Could you check a few things on this model? Use its own coordinates, in mm. A direction names the side the tool comes from. Round coordinates to 2 decimals unless told otherwise and drop trailing zeros. Write each loop counter-clockwise with the first axis right and the second up, starting at its lowest first coordinate (ties: lowest second). Pieces come first, ordered by that corner, then holes. Notation, with made-up numbers: M 51.5,-30 L 74.5,-30 A14 cw 74.5,-23 Z; hole C 60,51.5 d7. An arc over 180 degrees is marked long. One line per item, written item: value. Start each with the question number.
(1) If I drill on L1, parallel to Z at x = 8.89, y = 5; L2, parallel to Z at x = -0.5, y = 2.5; L3, parallel to Z at x = -19, y = 4.75, over which ranges is the centre line in solid material (lowest first)?
(2) I want a section at A-A on x = 0. Please give me the cut outline in (y, z).
(3) I want a section at B-B on z = 0. Please give me the cut outline in (x, y).
(4) I want a section at D-D on x = 5.5. Please give me the cut outline in (y, z), and give its area (3 significant figures).
(5) Which directions (+Z, -Z, +X, -X, +Y, -Y) give clear straight access to the entire face, cutting with the end or side of a thin tool? Please do faces 5 (the face through (-0.73, 3.13, -4.94)), 6 (the face through (15, 3, 15)), 7 (the face through (-20.047, 3.131, -5.372)).
(6) I'm going to push flat-ended pins straight in: pin 1 Ø2 at (y, z) = (2.5, 15) entering from +X; pin 2 Ø2 at (y, z) = (2.5, -13) entering from +X. Where does each tip first touch, or does it pass through?
(7) Thinking about a two-plate mould opening in X: for faces 1 (the face through (-9.06, 3.13, -15.3)), 2 (the face through (11.98, 3.13, 20.58)), 3 (the face through (2, 0, 0)), 4 (the face through (-23.812, 3.131, 0.087)), which applies, released by +X, released by -X, zero draft, split by the parting line, or undercut?
(8) I want a section at C-C on y = 5.25. Count the separate pieces of the cut face and the enclosed holes in it, and give its area (3 significant figures).
Autodesk Inventor part; units mm, degrees
ref_plane "YZ Plane" through (0, 0, 0) normal (1, 0, 0) x (0, 1, 0)
ref_plane "XZ Plane" through (0, 0, 0) normal (0, 1, 0) x (-1, 0, 0)
ref_plane "XY Plane" through (0, 0, 0) normal (0, 0, 1) x (1, 0, 0)
sketch "Sketch1" plane through (0, 0, 0) normal (0, 1, 0) x (-1, 0, 0)
  line L0 (17.1742, 4.6018) -> (23.0011, 6.1631)
  line L1 (17.1742, -4.6018) -> (23.0011, -6.1631)
  circle A0 centre (17.78, 0) radius 1.651
  line L2 (-12.5724, 12.5724) -> (-16.838, 16.838)
  line L3 (-4.6018, 17.1742) -> (-6.1631, 23.0011)
  circle A1 centre (-8.89, 15.3979) radius 1.651
  line L4 (-4.6018, -17.1742) -> (-6.1631, -23.0011)
  line L5 (-12.5724, -12.5724) -> (-16.838, -16.838)
  circle A2 centre (-8.89, -15.3979) radius 1.651
  arc A3 (-6.1631, 23.0011) -> (-16.838, 16.838) centre (0, 0) ccw
  arc A4 (-16.838, -16.838) -> (-6.1631, -23.0011) centre (0, 0) ccw
  arc A5 (23.0011, -6.1631) -> (23.0011, 6.1631) centre (0, 0) ccw
  arc A6 (-12.5724, 12.5724) -> (-12.5724, -12.5724) centre (0, 0) ccw
  arc A7 (-4.6018, -17.1742) -> (17.1742, -4.6018) centre (0, 0) ccw
  arc A8 (17.1742, 4.6018) -> (-4.6018, 17.1742) centre (0, 0) ccw
  circle A9 centre (6.35, 0) radius 1.5875
  circle A10 centre (0, 6.35) radius 1.5875
  circle A11 centre (-6.35, 0) radius 1.5875
  circle A12 centre (0, -6.35) radius 1.5875
  dimension "d3" = 3.302
  dimension "d9" = 3.175
  dimension "d12" = 360
  dimension "d15" = 6.35
extrude "Extrusion1" add sketch "Sketch1" along normal blind 6.35
properties part number "Hub_Adapter_Acryllic"
Found:
1. L1: z = -22.09 to -17.05, -13.75 to 13.75, 17.05 to 22.09
1. L2: z = -17.77 to -7.86, -4.84 to 4.84, 7.86 to 17.77
1. L3: z = -5.09 to -1.11, 1.11 to 5.09
2. outline: M 0,-17.78 L 6.35,-17.78 L 6.35,-7.94 L 0,-7.94 Z; M 0,-4.76 L 6.35,-4.76 L 6.35,4.76 L 0,4.76 Z; M 0,7.94 L 6.35,7.94 L 6.35,17.78 L 0,17.78 Z
3. outline: M -23.81,0 L -19.43,0 L -19.43,6.35 L -23.81,6.35 Z; M -16.13,0 L -7.94,0 L -7.94,6.35 L -16.13,6.35 Z; M -4.76,0 L 4.76,0 L 4.76,6.35 L -4.76,6.35 Z; M 7.94,0 L 17.78,0 L 17.78,6.35 L 7.94,6.35 Z
4. outline: M 0,-20.53 L 6.35,-20.53 L 6.35,-1.34 L 0,-1.34 Z; M 0,1.34 L 6.35,1.34 L 6.35,20.53 L 0,20.53 Z
4. area: 244 mm²
5. face 5: +Y, -Y
5. face 6: +X, +Y, -Y
5. face 7: -Z, +Y, -Y
6. pin 1: stops at x = 16
6. pin 2: stops at x = 14
7. face 1: undercut
7. face 2: released by +X
7. face 3: zero draft
7. face 4: released by -X
8. separate pieces: 1
8. enclosed holes: 7
8. area: 1,130 mm²
